Work out the finished part from the listing and answer in its coordinate system (mm). A direction names the side the tool comes from. Round coordinates to 2 decimals unless told otherwise and drop trailing zeros. Write each loop counter-clockwise with the first axis right and the second up, starting at its lowest first coordinate (ties: lowest second). Pieces come first, ordered by that corner, then holes.
1. Find section A-A (x = 1.25). Write down the section's boundary in (y, z).
2. Straight lines are drawn through the part: probe 1 along Z at (x, y) = (-2.55, -1); probe 2 along X at (y, z) = (-2.5, -0.15); probe 3 along Y at (x, z) = (0.85, 0.55). For each, find the intervals that lie inside material, in ascending order.
3. Flat-ended cylindrical pins translate along their axes: pin 1 Ø1.1 at (y, z) = (-2, 2.5) entering from +X; pin 2 Ø2 at (y, z) = (-2.5, 1.5) entering from -X; pin 3 Ø0.6 at (y, z) = (-1, 3) entering from -X. Find the tip coordinate at first contact, or state that the pin passes through.
4. Find section C-C (y = -2.5). Write down the section's boundary in (x, z), and give its area (3 significant figures).
5. A tool of negligible diameter and unlimited length cuts with its end or side. For faces 1 (the face through (0.961, -2, 1)), 2 (the face through (1.5, -1.9, 3.57)), 3 (the face through (-0.5, -1.8, -1.5)), from which of +Z, -Z, +X, -X, +Y, -Y can it reach the whole face along a straight path? Write none if from no direction.
```python
from build123d import *

# Parameters (mm, degrees)
SKETCH_3_W           = 3
SKETCH_3_H           = 6
EXTRUDE_2_DEPTH      = 3.5
SKETCH_4_OUTSIDE_W   = 6.514
SKETCH_4_OUTSIDE_H   = 9.514
SKETCH_4_OUTSIDE_W_2 = 1.417406922
SKETCH_4_OUTSIDE_H_2 = 3.080497711
CUT_EXTRUDE_1_DEPTH  = 0.8
SKETCH_9_W           = 3
SKETCH_9_H           = 6
EXTRUDE_5_DEPTH      = 1.5
FILLET_2_R           = 1
SKETCH_6_W           = 0.611138618
SKETCH_6_H           = 5.948224028
EXTRUDE_3_DEPTH      = 0.8
SKETCH_8_W           = 0.619217593
SKETCH_8_H           = 6
EXTRUDE_4_DEPTH      = 0.8
SKETCH_10_W          = 2.94488386
SKETCH_10_H          = 5.934698602
EXTRUDE_6_DEPTH      = 2
SKETCH_11_W          = 3
SKETCH_11_H          = 6
EXTRUDE_7_DEPTH      = 1.5
SKETCH_12_W          = 0.7
SKETCH_12_H          = 6
EXTRUDE_8_DEPTH      = 1.5
SKETCH_13_W          = 0.6302849
SKETCH_13_H          = 6
EXTRUDE_9_DEPTH      = 1.5
SKETCH_14_W          = 0.6302849
SKETCH_14_H          = 6
CUT_EXTRUDE_2_DEPTH  = 0.5
SKETCH_15_W          = 0.7
SKETCH_15_H          = 6
CUT_EXTRUDE_3_DEPTH  = 0.5
SKETCH_16_W          = 5
SKETCH_16_H          = 0.6302849
EXTRUDE_10_DEPTH     = 1
SKETCH_17_W          = 5
SKETCH_17_H          = 0.7
EXTRUDE_11_DEPTH     = 1
SKETCH_18_W          = 5
SKETCH_18_H          = 0.6302849
CUT_EXTRUDE_4_DEPTH  = 1
SKETCH_19_W          = 5
SKETCH_19_H          = 0.7
CUT_EXTRUDE_5_DEPTH  = 1


with BuildPart() as part:
    # 草图3 → 凸台-拉伸2 (new body)
    with BuildSketch(Plane.XY):
        with Locations((-0.538539978, -1.817017803)):
            Rectangle(SKETCH_3_W, SKETCH_3_H)
    extrude(amount=EXTRUDE_2_DEPTH)

    # 草图4 outside → 切除-拉伸1 (cut)
    with BuildSketch(Plane.XY.offset(3.5)):
        with Locations((-0.539, -1.817)):
            Rectangle(SKETCH_4_OUTSIDE_W, SKETCH_4_OUTSIDE_H)
        with Locations((-0.530790021, -1.736698078)):
            Rectangle(SKETCH_4_OUTSIDE_W_2, SKETCH_4_OUTSIDE_H_2, mode=Mode.SUBTRACT)
    extrude(amount=-CUT_EXTRUDE_1_DEPTH, mode=Mode.SUBTRACT)

    # 草图9 → 凸台-拉伸5 (add)
    with BuildSketch(Plane(origin=(0, 0, 0), x_dir=(-1, 0, 0), z_dir=(0, 0, -1))):
        with Locations((0.538539978, -1.817017803)):
            Rectangle(SKETCH_9_W, SKETCH_9_H)
    extrude(amount=EXTRUDE_5_DEPTH)

    # 圆角2
    fillet_2_edges = [part.edges().sort_by_distance(p)[0] for p in [
        (0.961460022, -1.817017803, -1.5),
        (-0.538539978, -4.817017803, -1.5),
        (-2.038539978, -1.817017803, -1.5),
        (-0.538539978, 1.182982197, -1.5),
    ]]
    fillet(fillet_2_edges, radius=FILLET_2_R)

    # 草图6 → 凸台-拉伸3 (add)
    with BuildSketch(Plane.ZY.offset(2.038539978)):
        with Locations((1.892599011, -1.842905789)):
            Rectangle(SKETCH_6_W, SKETCH_6_H)
    extrude(amount=EXTRUDE_3_DEPTH)

    # 草图8 → 凸台-拉伸4 (add)
    with BuildSketch(Plane(origin=(0.961460022, 0, 0), x_dir=(0, 0, -1), z_dir=(1, 0, 0))):
        with Locations((-1.93059109, -1.817017803)):
            Rectangle(SKETCH_8_W, SKETCH_8_H)
    extrude(amount=EXTRUDE_4_DEPTH)

    # 草图10 → 凸台-拉伸6 (add)
    with BuildSketch(Plane.XY.offset(3.5)):
        with Locations((-0.608169547, -1.884686131)):
            Rectangle(SKETCH_10_W, SKETCH_10_H)
    extrude(amount=-EXTRUDE_6_DEPTH)

    # 草图11 → 凸台-拉伸7 (add)
    with BuildSketch(Plane.XY.offset(2.7)):
        with Locations((-0.538539978, -1.817017803)):
            Rectangle(SKETCH_11_W, SKETCH_11_H)
    extrude(amount=EXTRUDE_7_DEPTH)

    # 草图12 → 凸台-拉伸8 (add)
    with BuildSketch(Plane.ZY.offset(2.038539978)):
        with Locations((3.85, -1.817017803)):
            Rectangle(SKETCH_12_W, SKETCH_12_H)
    extrude(amount=EXTRUDE_8_DEPTH)

    # 草图13 → 凸台-拉伸9 (add)
    with BuildSketch(Plane(origin=(0.961460022, 0, 0), x_dir=(0, 0, -1), z_dir=(1, 0, 0))):
        with Locations((-3.88485755, -1.817017803)):
            Rectangle(SKETCH_13_W, SKETCH_13_H)
    extrude(amount=EXTRUDE_9_DEPTH)

    # 草图14 → 切除-拉伸2 (cut)
    with BuildSketch(Plane(origin=(2.461460022, 0, 0), x_dir=(0, 0, -1), z_dir=(1, 0, 0))):
        with Locations((-3.88485755, -1.817017803)):
            Rectangle(SKETCH_14_W, SKETCH_14_H)
    extrude(amount=-CUT_EXTRUDE_2_DEPTH, mode=Mode.SUBTRACT)

    # 草图15 → 切除-拉伸3 (cut)
    with BuildSketch(Plane.ZY.offset(3.538539978)):
        with Locations((3.85, -1.817017803)):
            Rectangle(SKETCH_15_W, SKETCH_15_H)
    extrude(amount=-CUT_EXTRUDE_3_DEPTH, mode=Mode.SUBTRACT)

    # 草图16 → 凸台-拉伸10 (add)
    with BuildSketch(Plane(origin=(0, 1.182982197, 0), x_dir=(1, 0, 0), z_dir=(0, 1, 0))):
        with Locations((-0.538539978, -3.88485755)):
            Rectangle(SKETCH_16_W, SKETCH_16_H)
    extrude(amount=EXTRUDE_10_DEPTH)

    # 草图17 → 凸台-拉伸11 (add)
    with BuildSketch(Plane.XZ.offset(4.817017803)):
        with Locations((-0.538539978, 3.85)):
            Rectangle(SKETCH_17_W, SKETCH_17_H)
    extrude(amount=EXTRUDE_11_DEPTH)

    # 草图18 → 切除-拉伸4 (cut)
    with BuildSketch(Plane(origin=(0, 2.182982197, 0), x_dir=(1, 0, 0), z_dir=(0, 1, 0))):
        with Locations((-0.538539978, -3.88485755)):
            Rectangle(SKETCH_18_W, SKETCH_18_H)
    extrude(amount=-CUT_EXTRUDE_4_DEPTH, mode=Mode.SUBTRACT)

    # 草图19 → 切除-拉伸5 (cut)
    with BuildSketch(Plane.XZ.offset(5.817017803)):
        with Locations((-0.538539978, 3.85)):
            Rectangle(SKETCH_19_W, SKETCH_19_H)
    extrude(amount=-CUT_EXTRUDE_5_DEPTH, mode=Mode.SUBTRACT)


solid = part.part
```
Worked answers:
1. outline: (-4.82, 1.62) - (1.18, 1.62) - (1.18, 2.24) - (-4.82, 2.24) - close; (-4.82, 3.57) - (1.18, 3.57) - (1.18, 4.2) - (-4.82, 4.2) - close
2. probe 1: z = 1.59 to 2.2, 3.5 to 4.2
2. probe 2: x = -2.04 to 0.96
2. probe 3: y = -4.82 to 1.18
3. pin 1: stops at x = 1.76
3. pin 2: stops at x = -2.84
3. pin 3: stops at x = -2.08
4. outline: (-3.04, 3.5) - (-2.08, 3.5) - (-2.08, 2.2) - (-2.84, 2.2) - (-2.84, 1.59) - (-2.08, 1.59) - (-2.08, 1.5) - (-2.04, 1.5) - (-2.04, -0.5) arc R1 ccw to (-1.04, -1.5) - (-0.04, -1.5) arc R1 ccw to (0.96, -0.5) - (0.96, 1.62) - (1.76, 1.62) - (1.76, 2.24) - (0.96, 2.24) - (0.96, 3.57) - (1.96, 3.57) - (1.96, 4.2) - (-3.04, 4.2) - close
4. area: 19.0 mm2
5. face 1: -Z, +X, +Y, -Y
5. face 2: +X, +Y, -Y
5. face 3: -Z, +X, -X, +Y, -Y
